from build123d import *

# Parameters (mm, degrees)
F0_W      = 304.8
F0_H      = 152.4
F1_DEPTH  = 4.4958
F2_R      = 5.08
F3_R      = 4.8895
F4_DEPTH  = 4.4968
F5_R      = 11.1125
F6_DEPTH  = 4.4968
F7_R      = 19.05
F8_DEPTH  = 4.4968
F9_R      = 4.8895
F10_DEPTH = 4.4968


with BuildPart() as f1:
    # F0 (on Top) → F1 (new body)
    with BuildSketch(Plane.XY):
        Rectangle(F0_W, F0_H)
    extrude(amount=F1_DEPTH)

    # F2
    f2_edges = [f1.edges().sort_by_distance(p)[0] for p in [
        (-152.4, 76.2, 2.2479),
        (-152.4, -76.2, 2.2479),
        (152.4, -76.2, 2.2479),
        (152.4, 76.2, 2.2479),
    ]]
    fillet(f2_edges, radius=F2_R)

    # F3 (on face) → F4 (cut, through all)
    with BuildSketch(Plane.XY.offset(4.4958)):
        with Locations((-144.3355, 68.1355)):
            Circle(F3_R)
        with Locations((-144.3355, -68.1355)):
            Circle(F3_R)
        with Locations((144.3355, -68.1355)):
            Circle(F3_R)
        with Locations((144.3355, 68.1355)):
            Circle(F3_R)
    extrude(amount=-F4_DEPTH, mode=Mode.SUBTRACT)

    # F5 (on face) → F6 (cut, through all)
    with BuildSketch(Plane.XY.offset(4.4958)):
        with Locations((-106.3625, 52.3875)):
            Circle(F5_R)
        with Locations((-134.9375, 52.3875)):
            Circle(F5_R)
        with Locations((-134.9375, 17.4625)):
            Circle(F5_R)
        with Locations((-106.3625, 17.467218)):
            Circle(F5_R)
        with Locations((-134.9375, -17.4625)):
            Circle(F5_R)
        with Locations((-106.3625, -17.4625)):
            Circle(F5_R)
        with Locations((-134.9375, -52.3875)):
            Circle(F5_R)
        with Locations((-106.3625, -52.3875)):
            Circle(F5_R)
    extrude(amount=-F6_DEPTH, mode=Mode.SUBTRACT)

    # F7 (on face) → F8 (cut, through all)
    with BuildSketch(Plane.XY.offset(4.4958)):
        with Locations((120.65, 44.45)):
            Circle(F7_R)
        with Locations((120.65, 0)):
            Circle(F7_R)
        with Locations((120.65, -44.45)):
            Circle(F7_R)
    extrude(amount=-F8_DEPTH, mode=Mode.SUBTRACT)

    # F9 (on face) → F10 (cut, through all)
    with BuildSketch(Plane.XY.offset(4.4958)):
        with Locations((-93.5355, -64.9605)):
            Circle(F9_R)
        with Locations((93.5355, -64.9605)):
            Circle(F9_R)
    extrude(amount=-F10_DEPTH, mode=Mode.SUBTRACT)


solid = f1.part
CAD build for the part. Positions are in the model's coordinates, mm. Coordinates: 2 decimals unless noted, no trailing zeros. Order: outer loops, then holes, each group sorted by start corner. A loop starts at its lowest first (then second) coordinate and runs counter-clockwise, first axis right, second up.
Item 1: Band-saw the part on C-C on y = 44.45. List the corners of the cut face in (x, z), plus the area to 3 significant figures.
Check sheet entries:
outline: (-152.4, 0) - (-142.71, 0) - (-142.71, 4.5) - (-152.4, 4.5) - close; (-127.16, 0) - (-114.14, 0) - (-114.14, 4.5) - (-127.16, 4.5) - close; (-98.59, 0) - (101.6, 0) - (101.6, 4.5) - (-98.59, 4.5) - close; (139.7, 0) - (152.4, 0) - (152.4, 4.5) - (139.7, 4.5) - close
area: 1,060 mm2
Item 2: Band-saw the part on A-A on x = 120.65. List the corners of the cut face in (y, z).
Check sheet entries:
outline: (-76.2, 0) - (-63.5, 0) - (-63.5, 4.5) - (-76.2, 4.5) - close; (-25.4, 0) - (-19.05, 0) - (-19.05, 4.5) - (-25.4, 4.5) - close; (19.05, 0) - (25.4, 0) - (25.4, 4.5) - (19.05, 4.5) - close; (63.5, 0) - (76.2, 0) - (76.2, 4.5) - (63.5, 4.5) - close
Item 3: Pin check, flat tip, straight feed: pin 1 Ø20 at (x, y) = (-134.94, -52.39) entering from +Z. Stop position of the tip, or through.
Check sheet entries:
pin 1: passes through
Item 4: Band-saw the part on D-D on z = 2.2. Give the number of separate pieces and of enclosed holes in the cut face, plus the area to 3 significant figures.
Check sheet entries:
separate pieces: 1
enclosed holes: 17
area: 39,500 mm2
Item 5: Drill centre lines: L1, parallel to X at y = 57.5, z = 3.55; L2, parallel to X at y = 65.5, z = 1; L3, parallel to X at y = 47.5, z = 2.25. Where is each one in solid material? Low to high.
Check sheet entries:
L1: x = -152.4 to -144.8, -125.07 to -116.23, -96.5 to 106.77, 134.53 to 152.4
L2: x = -152.4 to -148.45, -140.22 to 140.22, 148.45 to 152.4
L3: x = -152.4 to -144.92, -124.96 to -116.34, -96.38 to 101.85, 139.45 to 152.4
Item 6: Two-plate mould, pull along Y, no slides. Class faces 1 (the face through (-2, 1, 4.496)), 2 (the face through (-148.216, -71.111, 2.279)): +Y half, -Y half, draft (parallel to the pull), parting line (faces both ways), or undercut.
Check sheet entries:
face 1: draft
face 2: undercut
Item 7: Band-saw the part on B-B on y = 0. List the corners of the cut face in (x, z), plus the area to 3 significant figures.
Check sheet entries:
outline: (-152.4, 0) - (101.6, 0) - (101.6, 4.5) - (-152.4, 4.5) - close; (139.7, 0) - (152.4, 0) - (152.4, 4.5) - (139.7, 4.5) - close
area: 1,200 mm2
